Source: CAD feature listing. Evaluate the final solid. Frame: model axes, mm. Face numbers are marked on the shaded views. Give positions to 0.01 mm unless a question says otherwise; leave off trailing zeros. Write each loop counter-clockwise with the first axis right and the second up, starting at its lowest first coordinate (ties: lowest second). Pieces come first, ordered by that corner, then holes. Notation, with made-up numbers: (83, 55) -> (140, 55) arc R29 ccw to (140, 94) -> close; hole circle Ø9 at (63, 13). An arc over 180 degrees is marked (long way). Use one line per item in the form item = value. Start each with the question number.
(1) Cut plane C-C, the plane z = 1.55. Output: boundary loops of the cut face in (x, y).
(2) Draft query along X for the marked faces 1, 2 and 3. Return one class per face: pulls with the +X half, pulls with the -X half, needs draft (parallel to the pull), parting line crosses it, or undercut.
(3) Cut plane D-D, the plane y = 2.6. Output: boundary loops of the cut face in (x, z), and give its area (3 significant figures).
(4) Material intervals for line 1 along X through (y, z) = (3, 0.85); line 2 along X through (y, z) = (5, 1.75); line 3 along Y through (x, z) = (9, 0.8), sorted ascending. Write a range as from..to.
(5) First-contact query: P1, Ø1.2, axis at x = 28, y = 2.6, coming from the -Z side. Flat tip, straight axial feed; report the tip coordinate or a pass-through.
(6) Cut plane A-A, the plane x = 28. Output: boundary loops of the cut face in (y, z), and give its area (3 significant figures).
(7) Cut plane B-B, the plane y = 10. Output: boundary loops of the cut face in (x, z), and give its area (3 significant figures).
from build123d import *

# Parameters (mm, degrees)
F0_W        = 30.6
F0_H        = 15
F0_R        = 0.65
F1_DEPTH    = 2.4
F2_R        = 3
F3_SIZE     = 2
F4_T1_DEPTH = 158.1036606393
F5_T1_DEPTH = 13.1878115659
F6_R        = 1.5
F6_R_2      = 4
F6_R_3      = 2.5
F7_DEPTH    = 25


# Not quite as in the source:
# - a fillet or chamfer that OpenCascade refuses, or shapes differently, is made with other operations: its cross-section is extruded or revolved along the edge and cut away or added


with BuildPart() as f1:
    # F0 (on Top) → F1 (new body)
    with BuildSketch(Plane.XY):
        with Locations((15.3, 7.5)):
            Rectangle(F0_W, F0_H)
        with Locations((28, 2.6)):
            Circle(F0_R, mode=Mode.SUBTRACT)
    extrude(amount=F1_DEPTH)

    # F2
    f2_edges = [f1.edges().sort_by_distance(p)[0] for p in [
        (30.6, 0, 1.2),
    ]]
    fillet(f2_edges, radius=F2_R)

    # F3
    f3_edges = [f1.edges().sort_by_distance(p)[0] for p in [
        (0, 0, 1.2),
        (0, 15, 1.2),
    ]]
    chamfer(f3_edges, length=F3_SIZE)

    # F4: chamfer of 30 x 10 on 1 edges, made by hand

    # F4_s2 → F4_t1 (cut)
    with BuildSketch(Plane.XY.offset(-77.8518303197)):
        Polygon((30.6, 5), (0.6, 15), (30.6, 15), align=None)
    extrude(amount=F4_T1_DEPTH, mode=Mode.SUBTRACT)

    # F5: fillet of radius 3 on 1 edges, made by hand

    # F5_s2 → F5_t1 (cut)
    with BuildSketch(Plane.XY.offset(-5.3939057829)):
        with BuildLine():
            ThreePointArc((28.553156669, 5.6822811103), (29.9893960062, 4.6561608917), (30.6, 3))
            Line((30.6, 3), (30.6, 5))
            Line((30.6, 5), (28.553156669, 5.6822811103))
        make_face()
    extrude(amount=F5_T1_DEPTH, mode=Mode.SUBTRACT)

    # F6 (on face) → F7 (cut)
    with BuildSketch(Plane.XY.offset(2.4)):
        with Locations((3.5149192099, 10.3407332852)):
            Circle(F6_R)
        with Locations((9.5205735153, 5.6994225355)):
            Circle(F6_R_2)
        with Locations((18.6217441043, 4.476449427)):
            Circle(F6_R_3)
    extrude(amount=-F7_DEPTH, mode=Mode.SUBTRACT)


solid = f1.part
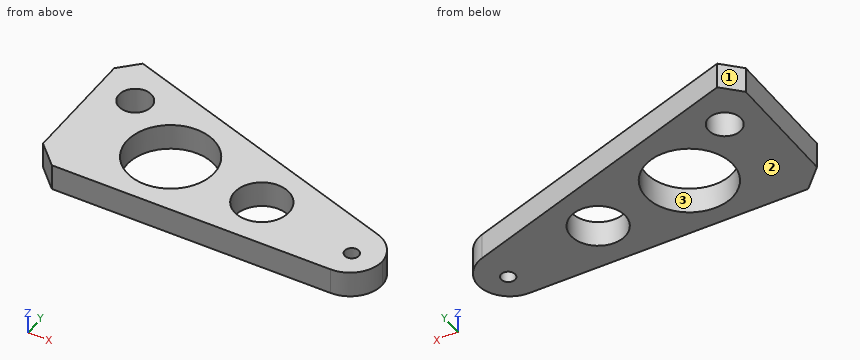
Geometry says:
q1.outline = (0, 2) -> (2, 0) -> (27.6, 0) arc R3 ccw to (30.6, 3) arc R3 ccw to (28.55, 5.68) -> (1.65, 14.65) -> (0, 13) -> close; hole circle Ø3 at (3.51, 10.34); hole circle Ø8 at (9.52, 5.7); hole circle Ø5 at (18.62, 4.48); hole circle Ø1.3 at (28, 2.6)
q2.face_1 = pulls with the -X half
q2.face_2 = needs draft
q2.face_3 = undercut
q3.outline = (0, 0) -> (6.99, 0) -> (6.99, 2.4) -> (0, 2.4) -> close; (12.05, 0) -> (16.97, 0) -> (16.97, 2.4) -> (12.05, 2.4) -> close; (20.27, 0) -> (27.35, 0) -> (27.35, 2.4) -> (20.27, 2.4) -> close; (28.65, 0) -> (30.57, 0) -> (30.57, 2.4) -> (28.65, 2.4) -> close
q3.area = 50.2 mm^2
q4.line_1 = 0..6.57, 12.47..16.6, 20.64..27.49, 28.51..30.6
q4.line_2 = 0..5.58, 13.46..16.18, 21.07..29.68
q4.line_3 = 0..1.73, 9.67..12.2
q5.P1 = through
q6.outline = (0.03, 0) -> (1.95, 0) -> (1.95, 2.4) -> (0.03, 2.4) -> close; (3.25, 0) -> (5.87, 0) -> (5.87, 2.4) -> (3.25, 2.4) -> close
q6.area = 10.9 mm^2
q7.outline = (0, 0) -> (2.05, 0) -> (2.05, 2.4) -> (0, 2.4) -> close; (4.98, 0) -> (15.6, 0) -> (15.6, 2.4) -> (4.98, 2.4) -> close
q7.area = 30.4 mm^2
